Check sheet for the modelled part. Datum: model origin and axes. Units: mm. Give positions to 0.01 mm unless a question says otherwise; leave off trailing zeros. Answer in a Markdown table with one row per item. Add a question column.
(1) Cross-section at A-A (z = 75.5). State how many separate pieces and enclosed holes the cut face has, then the cut area to 3 significant figures.
(2) Thickness scan on L1, parallel to Y at x = 0, z = 139.5; L2, parallel to Y at x = 3.25, z = -47.5; L3, parallel to X at y = -13, z = 262.5. Record the ranges inside material, lowest first. Write a range as [from, to].
(3) Release check for a two-part mould opening along Z. For faces 1 (the face through (-4, -5, -304.8)), 2 (the face through (-4, -5, 304.8)) record: released by +Z, released by -Z, zero draft, split by the parting line, or undercut.
(4) Go/stop test with flat-tipped pins: pin 1 (5 mm diameter, centred on y = -4.5, z = -190.5, fed in from +X); pin 2 (1.8 mm diameter, centred on y = 10.5, z = -1, fed in from +X); pin 3 (2.5 mm diameter, centred on x = 0, y = -10, fed in from +Z); pin 4 (0.7 mm diameter, centred on y = 10.5, z = 68.5, fed in from -X). Record where each tip stops, or that it passes through.
```python
from build123d import *

# Parameters (mm, degrees)
SKETCH3_R           = 2.15
BOSS_EXTRUDE1_DEPTH = 304.8
CIRPATTERN1_COUNT   = 2


with BuildPart() as part:
    # Sketch3 → Boss-Extrude1 (new, symmetric)
    with BuildSketch(Plane.XY):
        with BuildLine():
            Line((-8.30911066, 7.475083014), (-9.008684239, 7.499512662))
            ThreePointArc((-9.008684239, 7.499512662), (-9.582202525, 7.285082961), (-9.836116498, 6.727919597))
            Line((-9.836116498, 6.727919597), (-9.986803685, 2.412803152))
            ThreePointArc((-9.986803685, 2.412803152), (-9.995837451, 2.069746735), (-9.99898368, 1.726585818))
            Line((-9.99898368, 1.726585818), (-10, 0))
            Line((-10, 0), (-7.916458339, 0))
            ThreePointArc((-7.916458339, 0), (-7.764217404, 0.765366865), (-7.330671901, 1.414213562))
            Line((-7.330671901, 1.414213562), (-3.22356512, 5.521320344))
            ThreePointArc((-3.22356512, 5.521320344), (-2.250295073, 6.171638598), (-1.102244776, 6.4))
            Line((-1.102244776, 6.4), (1.102244776, 6.4))
            ThreePointArc((1.102244776, 6.4), (2.250295073, 6.171638598), (3.22356512, 5.521320344))
            Line((3.22356512, 5.521320344), (7.330671901, 1.414213562))
            ThreePointArc((7.330671901, 1.414213562), (7.764217404, 0.765366865), (7.916458339, 0))
            Line((7.916458339, 0), (10, 0))
            Line((10, 0), (9.99898368, 1.726585818))
            ThreePointArc((9.99898368, 1.726585818), (9.995837451, 2.069746735), (9.986803685, 2.412803152))
            Line((9.986803685, 2.412803152), (9.836116498, 6.727919597))
            ThreePointArc((9.836116498, 6.727919597), (9.582202525, 7.285082961), (9.008684239, 7.499512662))
            Line((9.008684239, 7.499512662), (8.30911066, 7.475083014))
            ThreePointArc((8.30911066, 7.475083014), (8.100174399, 7.379865274), (8.019763261, 7.164795917))
            Line((8.019763261, 7.164795917), (8.093719461, 5.046967452))
            ThreePointArc((8.093719461, 5.046967452), (7.631170264, 4.313871343), (6.779559917, 4.47555462))
            Line((6.779559917, 4.47555462), (4.478679656, 6.77643488))
            ThreePointArc((4.478679656, 6.77643488), (3.828361402, 7.749704927), (3.6, 8.897755224))
            Line((3.6, 8.897755224), (3.6, 11.102244776))
            ThreePointArc((3.6, 11.102244776), (3.828361402, 12.250295073), (4.478679656, 13.22356512))
            Line((4.478679656, 13.22356512), (6.779559917, 15.52444538))
            ThreePointArc((6.779559917, 15.52444538), (7.631170264, 15.686128657), (8.093719461, 14.953032548))
            Line((8.093719461, 14.953032548), (8.019763261, 12.835204083))
            ThreePointArc((8.019763261, 12.835204083), (8.100174399, 12.620134726), (8.30911066, 12.524916986))
            Line((8.30911066, 12.524916986), (9.008684239, 12.500487338))
            ThreePointArc((9.008684239, 12.500487338), (9.582202525, 12.714917039), (9.836116498, 13.272080403))
            Line((9.836116498, 13.272080403), (9.998781654, 17.930201007))
            ThreePointArc((9.998781654, 17.930201007), (9.414213562, 19.414213562), (7.930201007, 19.998781654))
            Line((7.930201007, 19.998781654), (3.272080403, 19.836116498))
            ThreePointArc((3.272080403, 19.836116498), (2.714917039, 19.582202525), (2.500487338, 19.008684239))
            Line((2.500487338, 19.008684239), (2.524916986, 18.30911066))
            ThreePointArc((2.524916986, 18.30911066), (2.620134726, 18.100174399), (2.835204083, 18.019763261))
            Line((2.835204083, 18.019763261), (4.953032548, 18.093719461))
            ThreePointArc((4.953032548, 18.093719461), (5.686128657, 17.631170264), (5.52444538, 16.779559917))
            Line((5.52444538, 16.779559917), (3.22356512, 14.478679656))
            ThreePointArc((3.22356512, 14.478679656), (2.250295073, 13.828361402), (1.102244776, 13.6))
            Line((1.102244776, 13.6), (-1.102244776, 13.6))
            ThreePointArc((-1.102244776, 13.6), (-2.250295073, 13.828361402), (-3.22356512, 14.478679656))
            Line((-3.22356512, 14.478679656), (-5.52444538, 16.779559917))
            ThreePointArc((-5.52444538, 16.779559917), (-5.686128657, 17.631170264), (-4.953032548, 18.093719461))
            Line((-4.953032548, 18.093719461), (-2.835204083, 18.019763261))
            ThreePointArc((-2.835204083, 18.019763261), (-2.620134726, 18.100174399), (-2.524916986, 18.30911066))
            Line((-2.524916986, 18.30911066), (-2.500487338, 19.008684239))
            ThreePointArc((-2.500487338, 19.008684239), (-2.714917039, 19.582202525), (-3.272080403, 19.836116498))
            Line((-3.272080403, 19.836116498), (-7.930201007, 19.998781654))
            ThreePointArc((-7.930201007, 19.998781654), (-9.414213562, 19.414213562), (-9.998781654, 17.930201007))
            Line((-9.998781654, 17.930201007), (-9.836116498, 13.272080403))
            ThreePointArc((-9.836116498, 13.272080403), (-9.582202525, 12.714917039), (-9.008684239, 12.500487338))
            Line((-9.008684239, 12.500487338), (-8.30911066, 12.524916986))
            ThreePointArc((-8.30911066, 12.524916986), (-8.100174399, 12.620134726), (-8.019763261, 12.835204083))
            Line((-8.019763261, 12.835204083), (-8.093719461, 14.953032548))
            ThreePointArc((-8.093719461, 14.953032548), (-7.631170264, 15.686128657), (-6.779559917, 15.52444538))
            Line((-6.779559917, 15.52444538), (-4.478679656, 13.22356512))
            ThreePointArc((-4.478679656, 13.22356512), (-3.828361402, 12.250295073), (-3.6, 11.102244776))
            Line((-3.6, 11.102244776), (-3.6, 8.897755224))
            ThreePointArc((-3.6, 8.897755224), (-3.828361402, 7.749704927), (-4.478679656, 6.77643488))
            Line((-4.478679656, 6.77643488), (-6.779559917, 4.47555462))
            ThreePointArc((-6.779559917, 4.47555462), (-7.631170264, 4.313871343), (-8.093719461, 5.046967452))
            Line((-8.093719461, 5.046967452), (-8.019763261, 7.164795917))
            ThreePointArc((-8.019763261, 7.164795917), (-8.100174399, 7.379865274), (-8.30911066, 7.475083014))
        make_face()
        with Locations(Location((0, 10, 0), (0, 0, 180))):
            Circle(SKETCH3_R, mode=Mode.SUBTRACT)
    boss_extrude1 = extrude(amount=BOSS_EXTRUDE1_DEPTH, both=True)

    # CirPattern1: Boss-Extrude1 ×2 about axis
    cirpattern1_axis = Axis((0, 0, 0), (0, 0, 1))
    for i in range(1, CIRPATTERN1_COUNT):
        add(boss_extrude1.rotate(cirpattern1_axis, i * 360 / CIRPATTERN1_COUNT))


solid = part.part
```
Answer below:
| question | item | result |
|---|---|---|
| 1 | separate pieces | 1 |
| 1 | enclosed holes | 3 |
| 1 | area | 327 mm² |
| 2 | L1 | y = [-13.6, -12.15], [-7.85, -6.4], [6.4, 7.85], [12.15, 13.6] |
| 2 | L2 | y = [-19.84, -18.03], [-14.51, -5.49], [5.49, 14.51], [18.03, 19.84] |
| 2 | L3 | x = [-9.78, -8.03], [-4.28, 4.28], [8.03, 9.78] |
| 3 | face 1 | released by -Z |
| 3 | face 2 | released by +Z |
| 4 | pin 1 | stops at x = 10 |
| 4 | pin 2 | stops at x = 3.61 |
| 4 | pin 3 | passes through |
| 4 | pin 4 | stops at x = -3.6 |
